Part model, mm, in its own coordinate system. Round coordinates to 2 decimals unless told otherwise and drop trailing zeros. Order: outer loops, then holes, each group sorted by start corner. A loop starts at its lowest first (then second) coordinate and runs counter-clockwise, first axis right, second up. Notation, with made-up numbers: M -13.5,-16.75 L -8.5,-16.75 A14 ccw -8.5,-11.75 Z; hole C -31.75,-16 d2. An arc over 180 degrees is marked long. One line per question, with ' | ' between items.
Autodesk Inventor part; units mm, degrees
ref_plane "YZ Plane" through (0, 0, 0) normal (1, 0, 0) x (0, 1, 0)
ref_plane "XZ Plane" through (0, 0, 0) normal (0, 1, 0) x (-1, 0, 0)
ref_plane "XY Plane" through (0, 0, 0) normal (0, 0, 1) x (1, 0, 0)
sketch "Sketch1" plane through (0, 0, 0) normal (0, 0, 1) x (1, 0, 0)
  line L0 (0, 0) -> (190.5, 0)
  line L1 (190.5, 0) -> (190.5, 546.1)
  line L2 (190.5, 546.1) -> (0, 546.1)
  line L3 (0, 0) -> (0, 546.1) construction
  line L4 (0, 0) -> (-190.5, 0)
  line L5 (-190.5, 0) -> (-190.5, 546.1)
  line L6 (-190.5, 546.1) -> (0, 546.1)
  line L7 (-165.1, 25.4) -> (165.1, 25.4)
  line L8 (165.1, 25.4) -> (165.1, 520.7)
  line L9 (165.1, 520.7) -> (-165.1, 520.7)
  line L10 (-165.1, 520.7) -> (-165.1, 25.4)
  dimension "d1" = 546.1
  dimension "d2" = 381
  dimension "d3" = 25.4
  dimension "d4" = 25.4
  dimension "d5" = 25.4
  dimension "d6" = 25.4
extrude "Extrusion1" add sketch "Sketch1" along normal mid plane 25.4
properties part number "primate2ndStageForShortRobot"
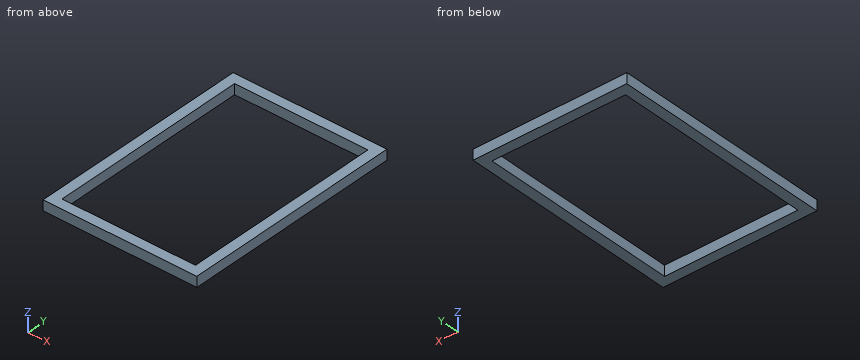
1) Saw through at B-B (x = -29.5). List the corners of the cut face in (y, z), plus the area to 3 significant figures.
The answers:
outline: M 0,-12.7 L 25.4,-12.7 L 25.4,12.7 L 0,12.7 Z; M 520.7,-12.7 L 546.1,-12.7 L 546.1,12.7 L 520.7,12.7 Z | area: 1,290 mm²
2) Saw through at C-C (z = -1.75). List the corners of the cut face in (x, y).
The answers:
outline: M -190.5,0 L 190.5,0 L 190.5,546.1 L -190.5,546.1 Z; hole M -165.1,25.4 L 165.1,25.4 L 165.1,520.7 L -165.1,520.7 Z
3) Saw through at A-A (y = 333). List the corners of the cut face in (x, z).
The answers:
outline: M -190.5,-12.7 L -165.1,-12.7 L -165.1,12.7 L -190.5,12.7 Z; M 165.1,-12.7 L 190.5,-12.7 L 190.5,12.7 L 165.1,12.7 Z
4) Probe line 1 (Y direction, x = -109.5, z = 6.75); line 2 (X direction, y = 331.5, z = 5). List the from-to ranges inside material, lowest first. Write a range as [from, to].
The answers:
line 1: y = [0, 25.4], [520.7, 546.1] | line 2: x = [-190.5, -165.1], [165.1, 190.5]
